Geometry: final body of the model. Coordinates: model frame, mm. Face numbers are marked on the shaded views. A direction names the side the tool comes from. Coordinates: 2 decimals unless noted, no trailing zeros. Order: outer loops, then holes, each group sorted by start corner. A loop starts at its lowest first (then second) coordinate and runs counter-clockwise, first axis right, second up. Notation, with made-up numbers: (42.5, 12.5) - (62.5, 12.5) arc R28 cw to (62.5, 44.5) - close; hole circle Ø9 at (36.25, 55). An arc over 180 degrees is marked (long way). Use a Markdown table: item, result. Add a question column.
```python
from build123d import *

# Parameters (mm, degrees)
SKETCH1_R           = 24
BOSS_EXTRUDE1_DEPTH = 11
SKETCH3_R           = 26
BOSS_EXTRUDE2_DEPTH = 2
SKETCH5_R           = 2.7
CUT_EXTRUDE1_DEPTH  = 46.033320997
SKETCH6_R           = 6.5
SKETCH6_R_2         = 2.7
BOSS_EXTRUDE3_DEPTH = 4


with BuildPart() as part:
    # Sketch1 → Boss-Extrude1 (new, symmetric)
    with BuildSketch(Plane.XY):
        Circle(SKETCH1_R)
    extrude(amount=BOSS_EXTRUDE1_DEPTH, both=True)

    # Sketch3 → Boss-Extrude2 (add)
    with BuildSketch(Plane.XY.offset(11)):
        Circle(SKETCH3_R)
    boss_extrude2 = extrude(amount=BOSS_EXTRUDE2_DEPTH)

    # Mirror1: Boss-Extrude2 across plane
    add(boss_extrude2.mirror(Plane.XY))

    # Sketch5 → Cut-Extrude1 (cut, through all)
    with BuildSketch(Plane.XY.offset(13)):
        Circle(SKETCH5_R)
    extrude(amount=-CUT_EXTRUDE1_DEPTH, mode=Mode.SUBTRACT)

    # Sketch6 → Boss-Extrude3 (add)
    with BuildSketch(Plane(origin=(0, 0, -13), x_dir=(-1, 0, 0), z_dir=(0, 0, -1))):
        Circle(SKETCH6_R)
        with Locations(Location((0, 0, 0), (0, 0, 180))):
            Circle(SKETCH6_R_2, mode=Mode.SUBTRACT)
    extrude(amount=BOSS_EXTRUDE3_DEPTH)


solid = part.part
```
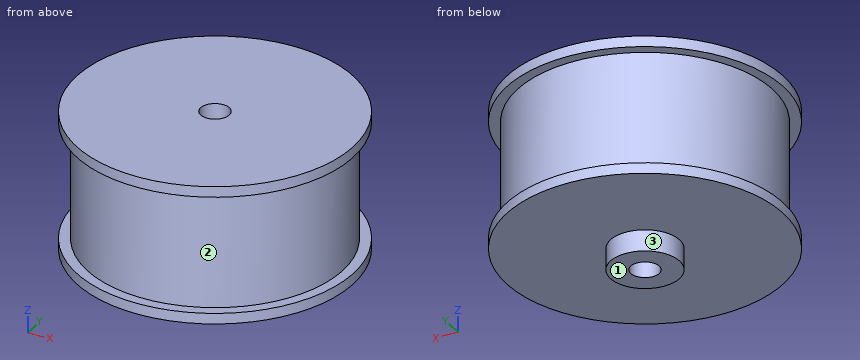
1) Pin query (flat end, axial travel): pin 1 (7 mm diameter, centred on x = 0, y = 0, fed in from +Z); pin 2 (12 mm diameter, centred on y = -1.5, z = 0, fed in from +X); pin 3 (8 mm diameter, centred on x = -10.5, y = -12, fed in from -Z); pin 4 (5 mm diameter, centred on x = 10, z = 4, fed in from +Y). Return the tip coordinate at first contact, or that it passes through.
2) Section C-C (z = 0.5). Return loops of the section in (x, y), then the cut area to 3 significant figures.
3) Ray query, line 1 along Y through (x, z) = (0, 5.5); line 2 along Z through (x, y) = (-24, -7); line 3 along Z through (x, y) = (3.5, -12). Return the intervals inside material, ascending.
4) Section A-A (y = 0). Return loops of the section in (x, z).
5) Section D-D (x = -10). Return loops of the section in (y, z).
6) Set-up query: the marked faces 1, 2 and 3. Return all of +Z, -Z, +X, -X, +Y, -Y with unobstructed straight access to the full face (end or side cutting, diameter ignored); none if empty.
Values follow:
| question | item | result |
|---|---|---|
| 1 | pin 1 | stops at z = 13 |
| 1 | pin 2 | stops at x = 24 |
| 1 | pin 3 | stops at z = -13 |
| 1 | pin 4 | stops at y = 22.8 |
| 2 | outline | circle Ø48 at (0, 0); hole circle Ø5.4 at (0, 0) |
| 2 | area | 1,790 mm² |
| 3 | line 1 | y = -24 to -2.7, 2.7 to 24 |
| 3 | line 2 | z = -13 to -11, 11 to 13 |
| 3 | line 3 | z = -13 to 13 |
| 4 | outline | (-26, -13) - (-6.5, -13) - (-6.5, -17) - (-2.7, -17) - (-2.7, 13) - (-26, 13) - (-26, 11) - (-24, 11) - (-24, -11) - (-26, -11) - close; (2.7, -17) - (6.5, -17) - (6.5, -13) - (26, -13) - (26, -11) - (24, -11) - (24, 11) - (26, 11) - (26, 13) - (2.7, 13) - close |
| 5 | outline | (-24, -13) - (24, -13) - (24, -11) - (21.82, -11) - (21.82, 11) - (24, 11) - (24, 13) - (-24, 13) - (-24, 11) - (-21.82, 11) - (-21.82, -11) - (-24, -11) - close |
| 6 | face 1 | -Z, +X, -X, +Y, -Y |
| 6 | face 2 | none |
| 6 | face 3 | -Z |
